The figure shows three views and two pictorial views of one solid part (mm, origin at its lowest corner). Answer the questions. A direction names the side the tool comes from. Coordinates: 2 decimals unless noted, no trailing zeros. Write each loop counter-clockwise with the first axis right and the second up, starting at its lowest first coordinate (ties: lowest second). Pieces come first, ordered by that corner, then holes.
Item 1: Each of these flat-tipped pins is pushed along its axis until it touches: P1, Ø17.5, axis at x = 81.5, y = 22.5, coming from the -Z side; P2, Ø1.3, axis at x = 23.5, y = 24.5, coming from the -Z side; P3, Ø3, axis at y = 29, z = 4, coming from the -X side. Where does it stop, or does it pass through?
Item 2: Section C-C (y = 18) is taken. Give the vertices of the cut face in (x, z), then the cut area to 3 significant figures.
Item 3: Determine the mould class of the marked faces 1, 2, 3 and 4 for opening direction Y: released by +Y, released by -Y, zero draft, split by the parting line, or undercut.
Item 4: A tool of negligible diameter and unlimited length cuts with its end or side. For the marked faces 5 and 6, from which of +Z, -Z, +X, -X, +Y, -Y can it reach the whole face along a straight path? Write none if from no direction.
Item 5: Straight lines are drawn through the part: probe 1 along Y at (x, z) = (49.5, 18.5); probe 2 along Z at (x, y) = (17, 22) (1 decimal); probe 3 along X at (y, z) = (11, 1.5). For each, find the intervals that lie inside material, in ascending order.
Item 6: Section D-D (y = 34.5) is taken. Give the vertices of the cut face in (x, z), then the cut area to 3 significant figures.
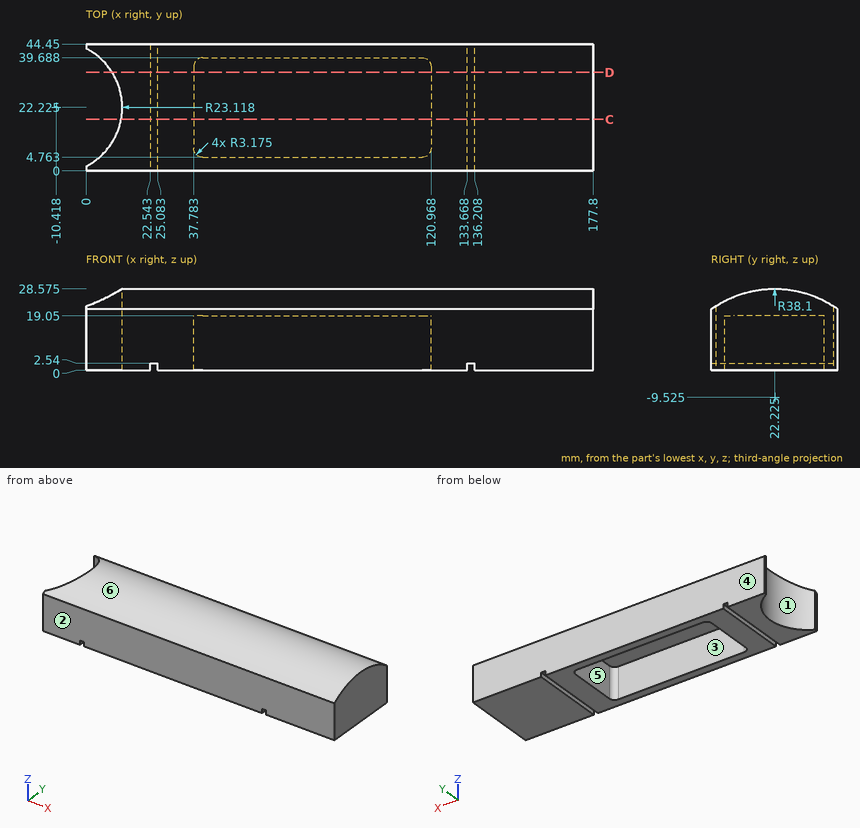
Established:
1. P1: stops at z = 19.05
1. P2: stops at z = 2.54
1. P3: stops at x = 11.17
2. outline: (12.31, 0) - (22.54, 0) - (22.54, 2.54) - (25.08, 2.54) - (25.08, 0) - (37.78, 0) - (37.78, 19.05) - (120.97, 19.05) - (120.97, 0) - (133.67, 0) - (133.67, 2.54) - (136.21, 2.54) - (136.21, 0) - (177.8, 0) - (177.8, 28.34) - (12.31, 28.34) - close
2. area: 3,090 mm2
3. face 1: undercut
3. face 2: released by -Y
3. face 3: undercut
3. face 4: released by +Y
4. face 5: -Z
4. face 6: +Z, +X, -X
5. probe 1: y = 0 to 4.76, 39.69 to 44.45
5. probe 2: z = 0 to 28.6
5. probe 3: x = 9.79 to 22.54, 25.08 to 37.78, 120.97 to 133.67, 136.21 to 177.8
6. outline: (9.17, 0) - (22.54, 0) - (22.54, 2.54) - (25.08, 2.54) - (25.08, 0) - (37.78, 0) - (37.78, 19.05) - (120.97, 19.05) - (120.97, 0) - (133.67, 0) - (133.67, 2.54) - (136.21, 2.54) - (136.21, 0) - (177.8, 0) - (177.8, 26.54) - (9.17, 26.54) - close
6. area: 2,880 mm2
